CAD build for the part. Positions are in the model's coordinates, mm. Coordinates: 2 decimals unless noted, no trailing zeros. Loops run counter-clockwise (first coordinate to the right, second up) from the corner with the lowest first, then second, coordinate; pieces in that order, holes last. Notation, with made-up numbers: (8.5, 72.5) -> (12.5, 72.5) arc R14 cw to (12.5, 80.5) -> close; hole circle Ø4 at (66, 68.5). An arc over 180 degrees is marked (long way). Write item = value, one per line. Start each with the question number.
(1) Flat gauge pins, fed straight in: P1, Ø8, axis at x = 11, z = 73, coming from the -Y side (3 decimals); P2, Ø10, axis at y = 8, z = 47, coming from the -X side; P3, Ø1.5, axis at x = 11.5, z = 32, coming from the -Y side. Where does each tip first touch, or does it go through?
(2) Band-saw the part on B-B (z = 26.5). Write the cut outline in (x, y), and give its area (3 significant figures).
(3) Drill centre lines: line 1 (Y direction, x = 0, z = 63); line 2 (X direction, y = 0.5, z = 64); line 3 (Z direction, x = -9, y = 0.5). Where is each one in solid material? Low to high. Write a range as from..to.
(4) Pull direction X, two halves, no side cores. Call faces 1 (the face through (11.82, 3.72, 78.39)), 2 (the face through (0, 0, 0)), 3 (the face through (-4.336, -19.524, 42.398)): +X half, -X half, draft (parallel to the pull), parting line (faces both ways), or undercut.
```python
from build123d import *

# Parameters (mm, degrees)
F0_R     = 20
F1_DEPTH = 86
F2_T     = -8
F3_SIZE  = 7.99999


# Not quite as in the source:
# - a fillet or chamfer is up to 0.001 mm smaller than in the source, because OpenCascade refuses the exact size


with BuildPart() as f1:
    # F0 (on Top) → F1 (new body)
    with BuildSketch(Plane.XY):
        Circle(F0_R)
    extrude(amount=F1_DEPTH)

    # F2
    f2_openings = [f1.faces().sort_by_distance(p)[0] for p in [
        (0, 0, 86),
    ]]
    offset(amount=F2_T, openings=f2_openings)

    # F3 (size 8 in the source; OpenCascade refuses exactly that, so slightly less here)
    f3_edges = [f1.edges().sort_by_distance(p)[0] for p in [
        (-12, 0, 86),
    ]]
    chamfer(f3_edges, length=F3_SIZE)


solid = f1.part
```
Findings below:
q1.P1 = -18.735
q1.P2 = -19.77
q1.P3 = -16.87
q2.outline = circle Ø40 at (0, 0); hole circle Ø24 at (0, 0)
q2.area = 804 mm²
q3.line_1 = -20..-12, 12..20
q3.line_2 = -19.99..-11.99, 11.99..19.99
q3.line_3 = 0..8
q4.face_1 = undercut
q4.face_2 = draft
q4.face_3 = parting line
